from build123d import *

# Parameters (mm, degrees)
SKETCH1_R           = 63.5
BOSS_EXTRUDE1_DEPTH = 15.875
BOSS_EXTRUDE2_START = 93.472
SKETCH2_W           = 66.04
SKETCH2_H           = 94.996
SKETCH2_R           = 3.96875
BOSS_EXTRUDE2_DEPTH = 6.35
SKETCH3_W           = 17.145
SKETCH3_H           = 38.1
BOSS_EXTRUDE3_DEPTH = 112.522
FILLET1_R           = 19.05


with BuildPart() as part:
    # Sketch1 → Boss-Extrude1 (new, symmetric)
    with BuildSketch(Plane(origin=(0, 0, 0), x_dir=(0, 0, -1), z_dir=(1, 0, 0))):
        Circle(SKETCH1_R)
    extrude(amount=BOSS_EXTRUDE1_DEPTH, both=True)



with BuildPart() as body_2:
    # Sketch2 → Boss-Extrude2 (new body)
    with BuildSketch(Plane(origin=(0, 0, 0), x_dir=(1, 0, 0), z_dir=(0, 1, 0)).offset(BOSS_EXTRUDE2_START)):
        Rectangle(SKETCH2_W, SKETCH2_H)
        with Locations(Location((-22.86, 37.211, 0), (0, 0, 270))):
            Circle(SKETCH2_R, mode=Mode.SUBTRACT)
        with Locations(Location((22.86, 37.211, 0), (0, 0, 270))):
            Circle(SKETCH2_R, mode=Mode.SUBTRACT)
        with Locations(Location((22.86, -37.211, 0), (0, 0, 270))):
            Circle(SKETCH2_R, mode=Mode.SUBTRACT)
        with Locations(Location((-22.86, -37.211, 0), (0, 0, 270))):
            Circle(SKETCH2_R, mode=Mode.SUBTRACT)
    extrude(amount=-BOSS_EXTRUDE2_DEPTH)


with BuildPart() as part_1:
    add(part.part)

    add(body_2.part)  # Boss-Extrude3 merges body 2
    # Sketch3 → Boss-Extrude3 (add)
    with BuildSketch(Plane.XZ.offset(-87.122)):
        with Locations((-24.4475, 0)):
            Rectangle(SKETCH3_W, SKETCH3_H)
        with Locations((24.4475, 0)):
            Rectangle(SKETCH3_W, SKETCH3_H)
    extrude(amount=BOSS_EXTRUDE3_DEPTH)

    # Fillet1
    fillet1_edges = [part_1.edges().sort_by_distance(p)[0] for p in [
        (-24.4475, -25.4, -19.05),
        (-24.4475, -25.4, 19.05),
        (24.4475, -25.4, 19.05),
        (24.4475, -25.4, -19.05),
    ]]
    fillet(fillet1_edges, radius=FILLET1_R - 0.0001)  # a hair under: the kernel refuses the full size


solid = part_1.part
Build history of the part. All positions in model axes, mm. A direction names the side the tool comes from. Coordinates: 2 decimals unless noted, no trailing zeros. Write each loop counter-clockwise with the first axis right and the second up, starting at its lowest first coordinate (ties: lowest second). Pieces come first, ordered by that corner, then holes.
(1) Cut at A-A on x = -22.86. State how many separate pieces and enclosed holes the cut face has, and give its area (3 significant figures).
(2) Cut at C-C on y = 0. List the corners of the cut face in (x, z) (3 decimals).
(3) Drill centre lines: line 1 (X direction, y = 85, z = 1) (3 decimals); line 2 (Z direction, x = -22, y = 90); line 3 (Y direction, x = 29, z = 0). Where is each one in solid material? Low to high.
(4) 3-axis set-ups, long thin cutter, end or side, ignore diameter. For faces 1 (the flat face through (15.875, -28, 1)), 2 (the cylindrical face through (24.57, -19.67, -13.62)), 3 (the flat face through (-25, 41, -19.05)), 4 (the flat face through (0, 87.122, -1)), 5 (the cylindrical face through (24.57, -19.67, 13.62)): which of +Z, -Z, +X, -X, +Y, -Y reach the whole face in a straight line?
(5) Mould opens along X. For faces 6 (the flat face through (15.875, 74, 0)), 7 (the flat face through (-15.875, -28, 1)), 8 (the flat face through (33.02, 48, 1)), 9 (the flat face through (24, 41, 19.05)) say: pulls with the +X half, pulls with the -X half, needs draft (parallel to the pull), parting line crosses it, or undercut.
(6) Pin check, flat tips, straight feed: pin 1 Ø12 at (x, z) = (11, -43) entering from -Y; pin 2 Ø10.5 at (x, z) = (22.86, -37.211) entering from -Y; pin 3 Ø5 at (x, y) = (22, 31.5) entering from -Z. Stop position of each tip, or through.
(7) Cut at D-D on z = -35. List the corners of the cut face in (x, y) (3 decimals).
(8) Cut at B-B on x = 12. List the corners of the cut face in (y, z).
Working result:
1. separate pieces: 3
1. enclosed holes: 0
1. area: 4,630 mm2
2. outline: (-33.02, -19.05) - (-15.875, -19.05) - (-15.875, -63.5) - (15.875, -63.5) - (15.875, -19.05) - (33.02, -19.05) - (33.02, 19.05) - (15.875, 19.05) - (15.875, 63.5) - (-15.875, 63.5) - (-15.875, 19.05) - (-33.02, 19.05) - close
3. line 1: x = -33.02 to -15.875, 15.875 to 33.02
3. line 2: z = -47.5 to -41.09, -33.34 to 33.34, 41.09 to 47.5
3. line 3: y = -25.4 to 93.47
4. face 1: +X, -Y
4. face 2: -Z, +X, -Y
4. face 3: -Z, -X, -Y
4. face 4: none
4. face 5: +Z, +X, -Y
5. face 6: undercut
5. face 7: pulls with the -X half
5. face 8: pulls with the +X half
5. face 9: needs draft
6. pin 1: stops at y = -51.61
6. pin 2: stops at y = 87.12
6. pin 3: stops at z = -19.05
7. outline: (-33.02, 87.122) - (-26.156, 87.122) - (-26.156, 93.472) - (-33.02, 93.472) - close; (-19.564, 87.122) - (19.564, 87.122) - (19.564, 93.472) - (-19.564, 93.472) - close; (-15.875, -52.983) - (15.875, -52.983) - (15.875, 52.983) - (-15.875, 52.983) - close; (26.156, 87.122) - (33.02, 87.122) - (33.02, 93.472) - (26.156, 93.472) - close
8. outline: circle Ø127 at (0, 0); (87.12, -47.5) - (93.47, -47.5) - (93.47, 47.5) - (87.12, 47.5) - close
